from build123d import *

# Parameters (mm, degrees)
SKETCH1_R           = 3.5
BOSS_EXTRUDE1_DEPTH = 4
SKETCH2_R           = 1
SKETCH2_R_2         = 0.5
BOSS_EXTRUDE2_DEPTH = 1.5
SKETCH3_R           = 2.25
CUT_EXTRUDE1_DEPTH  = 1


with BuildPart() as part:
    # Sketch1 → Boss-Extrude1 (new body)
    with BuildSketch(Plane(origin=(0, 0, 0), x_dir=(1, 0, 0), z_dir=(0, 1, 0))):
        with Locations(Location((0, 0, 0), (0, 0, 270))):
            Circle(SKETCH1_R)
        with BuildLine():
            Line((2.392601601, 0.18830183), (2.492293334, 0.196147739))
            ThreePointArc((2.492293334, 0.196147739), (2.5, 0), (2.492293334, -0.196147739))
            Line((2.492293334, -0.196147739), (2.392601601, -0.18830183))
            ThreePointArc((2.392601601, -0.18830183), (2.383364297, -0.282089754), (2.370452017, -0.375442716))
            ThreePointArc((2.370452017, -0.375442716), (2.353884673, -0.468216773), (2.333687809, -0.560268873))
            Line((2.333687809, -0.560268873), (2.430924801, -0.58361341))
            ThreePointArc((2.430924801, -0.58361341), (2.377641291, -0.772542486), (2.309698831, -0.956708581))
            Line((2.309698831, -0.956708581), (2.217310878, -0.918440238))
            ThreePointArc((2.217310878, -0.918440238), (2.179543617, -1.00478337), (2.138415658, -1.089577199))
            ThreePointArc((2.138415658, -1.089577199), (2.093990417, -1.17269098), (2.046336394, -1.253996555))
            Line((2.046336394, -1.253996555), (2.131600411, -1.306246412))
            ThreePointArc((2.131600411, -1.306246412), (2.022542486, -1.469463131), (1.901014914, -1.623620121))
            Line((1.901014914, -1.623620121), (1.824974317, -1.558675316))
            ThreePointArc((1.824974317, -1.558675316), (1.762374023, -1.629121789), (1.697056275, -1.697056275))
            ThreePointArc((1.697056275, -1.697056275), (1.629121789, -1.762374023), (1.558675316, -1.824974317))
            Line((1.558675316, -1.824974317), (1.623620121, -1.901014914))
            ThreePointArc((1.623620121, -1.901014914), (1.469463131, -2.022542486), (1.306246412, -2.131600411))
            Line((1.306246412, -2.131600411), (1.253996555, -2.046336394))
            ThreePointArc((1.253996555, -2.046336394), (1.17269098, -2.093990417), (1.089577199, -2.138415658))
            ThreePointArc((1.089577199, -2.138415658), (1.00478337, -2.179543617), (0.918440238, -2.217310878))
            Line((0.918440238, -2.217310878), (0.956708581, -2.309698831))
            ThreePointArc((0.956708581, -2.309698831), (0.772542486, -2.377641291), (0.58361341, -2.430924801))
            Line((0.58361341, -2.430924801), (0.560268873, -2.333687809))
            ThreePointArc((0.560268873, -2.333687809), (0.468216773, -2.353884673), (0.375442716, -2.370452017))
            ThreePointArc((0.375442716, -2.370452017), (0.282089754, -2.383364297), (0.18830183, -2.392601601))
            Line((0.18830183, -2.392601601), (0.196147739, -2.492293334))
            ThreePointArc((0.196147739, -2.492293334), (0, -2.5), (-0.196147739, -2.492293334))
            Line((-0.196147739, -2.492293334), (-0.18830183, -2.392601601))
            ThreePointArc((-0.18830183, -2.392601601), (-0.282089754, -2.383364297), (-0.375442716, -2.370452017))
            ThreePointArc((-0.375442716, -2.370452017), (-0.468216773, -2.353884673), (-0.560268873, -2.333687809))
            Line((-0.560268873, -2.333687809), (-0.58361341, -2.430924801))
            ThreePointArc((-0.58361341, -2.430924801), (-0.772542486, -2.377641291), (-0.956708581, -2.309698831))
            Line((-0.956708581, -2.309698831), (-0.918440238, -2.217310878))
            ThreePointArc((-0.918440238, -2.217310878), (-1.00478337, -2.179543617), (-1.089577199, -2.138415658))
            ThreePointArc((-1.089577199, -2.138415658), (-1.17269098, -2.093990417), (-1.253996555, -2.046336394))
            Line((-1.253996555, -2.046336394), (-1.306246412, -2.131600411))
            ThreePointArc((-1.306246412, -2.131600411), (-1.469463131, -2.022542486), (-1.623620121, -1.901014914))
            Line((-1.623620121, -1.901014914), (-1.558675316, -1.824974317))
            ThreePointArc((-1.558675316, -1.824974317), (-1.629121789, -1.762374023), (-1.697056275, -1.697056275))
            ThreePointArc((-1.697056275, -1.697056275), (-1.762374023, -1.629121789), (-1.824974317, -1.558675316))
            Line((-1.824974317, -1.558675316), (-1.901014914, -1.623620121))
            ThreePointArc((-1.901014914, -1.623620121), (-2.022542486, -1.469463131), (-2.131600411, -1.306246412))
            Line((-2.131600411, -1.306246412), (-2.046336394, -1.253996555))
            ThreePointArc((-2.046336394, -1.253996555), (-2.093990417, -1.17269098), (-2.138415658, -1.089577199))
            ThreePointArc((-2.138415658, -1.089577199), (-2.179543617, -1.00478337), (-2.217310878, -0.918440238))
            Line((-2.217310878, -0.918440238), (-2.309698831, -0.956708581))
            ThreePointArc((-2.309698831, -0.956708581), (-2.377641291, -0.772542486), (-2.430924801, -0.58361341))
            Line((-2.430924801, -0.58361341), (-2.333687809, -0.560268873))
            ThreePointArc((-2.333687809, -0.560268873), (-2.353884673, -0.468216773), (-2.370452017, -0.375442716))
            ThreePointArc((-2.370452017, -0.375442716), (-2.383364297, -0.282089754), (-2.392601601, -0.18830183))
            Line((-2.392601601, -0.18830183), (-2.492293334, -0.196147739))
            ThreePointArc((-2.492293334, -0.196147739), (-2.5, 0), (-2.492293334, 0.196147739))
            Line((-2.492293334, 0.196147739), (-2.392601601, 0.18830183))
            ThreePointArc((-2.392601601, 0.18830183), (-2.383364297, 0.282089754), (-2.370452017, 0.375442716))
            ThreePointArc((-2.370452017, 0.375442716), (-2.353884673, 0.468216773), (-2.333687809, 0.560268873))
            Line((-2.333687809, 0.560268873), (-2.430924801, 0.58361341))
            ThreePointArc((-2.430924801, 0.58361341), (-2.377641291, 0.772542486), (-2.309698831, 0.956708581))
            Line((-2.309698831, 0.956708581), (-2.217310878, 0.918440238))
            ThreePointArc((-2.217310878, 0.918440238), (-2.179543617, 1.00478337), (-2.138415658, 1.089577199))
            ThreePointArc((-2.138415658, 1.089577199), (-2.093990417, 1.17269098), (-2.046336394, 1.253996555))
            Line((-2.046336394, 1.253996555), (-2.131600411, 1.306246412))
            ThreePointArc((-2.131600411, 1.306246412), (-2.022542486, 1.469463131), (-1.901014914, 1.623620121))
            Line((-1.901014914, 1.623620121), (-1.824974317, 1.558675316))
            ThreePointArc((-1.824974317, 1.558675316), (-1.762374023, 1.629121789), (-1.697056275, 1.697056275))
            ThreePointArc((-1.697056275, 1.697056275), (-1.629121789, 1.762374023), (-1.558675316, 1.824974317))
            Line((-1.558675316, 1.824974317), (-1.623620121, 1.901014914))
            ThreePointArc((-1.623620121, 1.901014914), (-1.469463131, 2.022542486), (-1.306246412, 2.131600411))
            Line((-1.306246412, 2.131600411), (-1.253996555, 2.046336394))
            ThreePointArc((-1.253996555, 2.046336394), (-1.17269098, 2.093990417), (-1.089577199, 2.138415658))
            ThreePointArc((-1.089577199, 2.138415658), (-1.00478337, 2.179543617), (-0.918440238, 2.217310878))
            Line((-0.918440238, 2.217310878), (-0.956708581, 2.309698831))
            ThreePointArc((-0.956708581, 2.309698831), (-0.772542486, 2.377641291), (-0.58361341, 2.430924801))
            Line((-0.58361341, 2.430924801), (-0.560268873, 2.333687809))
            ThreePointArc((-0.560268873, 2.333687809), (-0.468216773, 2.353884673), (-0.375442716, 2.370452017))
            ThreePointArc((-0.375442716, 2.370452017), (-0.282089754, 2.383364297), (-0.18830183, 2.392601601))
            Line((-0.18830183, 2.392601601), (-0.196147739, 2.492293334))
            ThreePointArc((-0.196147739, 2.492293334), (0, 2.5), (0.196147739, 2.492293334))
            Line((0.196147739, 2.492293334), (0.18830183, 2.392601601))
            ThreePointArc((0.18830183, 2.392601601), (0.282089754, 2.383364297), (0.375442716, 2.370452017))
            ThreePointArc((0.375442716, 2.370452017), (0.468216773, 2.353884673), (0.560268873, 2.333687809))
            Line((0.560268873, 2.333687809), (0.58361341, 2.430924801))
            ThreePointArc((0.58361341, 2.430924801), (0.772542486, 2.377641291), (0.956708581, 2.309698831))
            Line((0.956708581, 2.309698831), (0.918440238, 2.217310878))
            ThreePointArc((0.918440238, 2.217310878), (1.00478337, 2.179543617), (1.089577199, 2.138415658))
            ThreePointArc((1.089577199, 2.138415658), (1.17269098, 2.093990417), (1.253996555, 2.046336394))
            Line((1.253996555, 2.046336394), (1.306246412, 2.131600411))
            ThreePointArc((1.306246412, 2.131600411), (1.469463131, 2.022542486), (1.623620121, 1.901014914))
            Line((1.623620121, 1.901014914), (1.558675316, 1.824974317))
            ThreePointArc((1.558675316, 1.824974317), (1.629121789, 1.762374023), (1.697056275, 1.697056275))
            ThreePointArc((1.697056275, 1.697056275), (1.762374023, 1.629121789), (1.824974317, 1.558675316))
            Line((1.824974317, 1.558675316), (1.901014914, 1.623620121))
            ThreePointArc((1.901014914, 1.623620121), (2.022542486, 1.469463131), (2.131600411, 1.306246412))
            Line((2.131600411, 1.306246412), (2.046336394, 1.253996555))
            ThreePointArc((2.046336394, 1.253996555), (2.093990417, 1.17269098), (2.138415658, 1.089577199))
            ThreePointArc((2.138415658, 1.089577199), (2.179543617, 1.00478337), (2.217310878, 0.918440238))
            Line((2.217310878, 0.918440238), (2.309698831, 0.956708581))
            ThreePointArc((2.309698831, 0.956708581), (2.377641291, 0.772542486), (2.430924801, 0.58361341))
            Line((2.430924801, 0.58361341), (2.333687809, 0.560268873))
            ThreePointArc((2.333687809, 0.560268873), (2.353884673, 0.468216773), (2.370452017, 0.375442716))
            ThreePointArc((2.370452017, 0.375442716), (2.383364297, 0.282089754), (2.392601601, 0.18830183))
        make_face(mode=Mode.SUBTRACT)
    extrude(amount=BOSS_EXTRUDE1_DEPTH)

    # Sketch2 → Boss-Extrude2 (add)
    with BuildSketch(Plane.XZ):
        with BuildLine():
            Line((-14.214285714, 1.988487272), (-0.375, 3.479852727))
            ThreePointArc((-0.375, 3.479852727), (3.5, 0), (-0.375, -3.479852727))
            Line((-0.375, -3.479852727), (-14.214285714, -1.988487272))
            ThreePointArc((-14.214285714, -1.988487272), (-16, 0), (-14.214285714, 1.988487272))
        make_face()
        with Locations(Location((0, 0, 0), (0, 0, 270))):
            Circle(SKETCH2_R, mode=Mode.SUBTRACT)
        with Locations(Location((-14.667614311, 0, 0), (0, 0, 270))):
            Circle(SKETCH2_R_2, mode=Mode.SUBTRACT)
        with Locations(Location((-12.667614311, 0, 0), (0, 0, 270))):
            Circle(SKETCH2_R_2, mode=Mode.SUBTRACT)
        with Locations(Location((-10.667614311, 0, 0), (0, 0, 270))):
            Circle(SKETCH2_R_2, mode=Mode.SUBTRACT)
        with Locations(Location((-8.667614311, 0, 0), (0, 0, 270))):
            Circle(SKETCH2_R_2, mode=Mode.SUBTRACT)
        with Locations(Location((-6.667614311, 0, 0), (0, 0, 270))):
            Circle(SKETCH2_R_2, mode=Mode.SUBTRACT)
        with Locations(Location((-4.667614311, 0, 0), (0, 0, 270))):
            Circle(SKETCH2_R_2, mode=Mode.SUBTRACT)
    extrude(amount=-BOSS_EXTRUDE2_DEPTH)

    # Sketch3 → Cut-Extrude1 (cut)
    with BuildSketch(Plane(origin=(0, 0, 0), x_dir=(-1, 0, 0), z_dir=(0, -1, 0))):
        with Locations(Location((0, 0, 0), (0, 0, 90))):
            Circle(SKETCH3_R)
    extrude(amount=-CUT_EXTRUDE1_DEPTH, mode=Mode.SUBTRACT)


solid = part.part
Could you check a few things on this model? Use its own coordinates, in mm. A direction names the side the tool comes from. Coordinates: 2 decimals unless noted, no trailing zeros. Order: outer loops, then holes, each group sorted by start corner. A loop starts at its lowest first (then second) coordinate and runs counter-clockwise, first axis right, second up. Notation, with made-up numbers: (8, -8) -> (16, -8) arc R38 cw to (16, 31) -> close; hole circle Ø3 at (0.25, 27). An arc over 180 degrees is marked (long way). One line per item, written item: value. Start each with the question number.
1) Imagine slicing it at A-A on x = 0. List the corners of the cut face in (y, z) for me.
2) Imagine slicing it at D-D on z = 2.75. List the corners of the cut face in (x, y) for me, plus the area to 3 significant figures.
3) Imagine slicing it at B-B on y = 0.6. List the corners of the cut face in (x, z) for me (3 decimals).
4) We'd pull the mould along X, two halves only. Please class faces 4 (the flat face through (-6, 0, 0)), 5 (the flat face through (-7.392, 0.74, 2.724)), 6 (the cylindrical face through (-10.172, 0.74, 0.065)): +X half, -X half, draft (parallel to the pull), parting line (faces both ways), or undercut.
5) I'm going to push flat-ended pins straight in: pin 1 (3 mm diameter, centred on x = -12.5, z = -2, fed in from +Y); pin 2 (1 mm diameter, centred on y = 1.5, z = 2, fed in from +X); pin 3 (2 mm diameter, centred on x = 0.5, z = 0.5, fed in from -Y). Where does each tip first touch, or does it pass through?
6) Imagine slicing it at C-C on z = 0. Count the separate pieces of the cut face and the enclosed holes in it, plus the area to 4 significant figures.
7) If I drill on L1, parallel to Y at x = -8.5, z = -2.5; L2, parallel to Y at x = 1.75, z = 0.25; L3, parallel to Z at x = 2, y = 1.8, over which ranges is the centre line in solid material (lowest first)? Write a range as [from, to].
8) Which directions (+Z, -Z, +X, -X, +Y, -Y) give clear straight access to the entire face, cutting with the end or side of a thin tool? Please do faces 1 (the cylindrical face through (3.47, 2.42, -0.46)), 2 (the flat face through (-1, 1, 1)), 3 (the flat face through (-2, 4, 2)).
Answer list:
1. outline: (0, -3.5) -> (4, -3.5) -> (4, -2.5) -> (1.5, -2.5) -> (1.5, -1) -> (1, -1) -> (1, -2.25) -> (0, -2.25) -> close; (0, 2.25) -> (1, 2.25) -> (1, 1) -> (1.5, 1) -> (1.5, 2.5) -> (4, 2.5) -> (4, 3.5) -> (0, 3.5) -> close
2. outline: (-7.15, 0) -> (2.17, 0) -> (2.17, 4) -> (-2.17, 4) -> (-2.17, 1.5) -> (-7.15, 1.5) -> close
2. area: 24.8 mm2
3. outline: (-14.214, -1.988) -> (-0.375, -3.48) arc R3.5 ccw (long way) to (-0.375, 3.48) -> (-14.214, 1.988) arc R2 ccw to start; hole circle Ø1 at (-14.668, 0); hole circle Ø1 at (-12.668, 0); hole circle Ø1 at (-10.668, 0); hole circle Ø1 at (-8.668, 0); hole circle Ø1 at (-6.668, 0); hole circle Ø1 at (-4.668, 0); hole circle Ø4.5 at (0, 0)
4. face 4: draft
4. face 5: -X half
4. face 6: undercut
5. pin 1: stops at y = 1.5
5. pin 2: stops at x = 3.16
5. pin 3: stops at y = 1
6. separate pieces: 8
6. enclosed holes: 0
6. area: 19.75 mm2
7. L1: y = [0, 1.5]
7. L2: y = [1, 1.5]
7. L3: z = [-2.87, -1.5], [1.5, 2.87]
8. face 1: +Y
8. face 2: -Y
8. face 3: +Z, -Z, +X, -X, +Y
